from build123d import *

# Parameters (mm, degrees)
F0_R      = 73.025
F0_R_2    = 60.325
F1_DEPTH  = 69.85
F2_DEPTH  = 57.15
F3_SIZE   = 6.35
F4_DEPTH  = 12.7
F4_FACE_R = 73.025
F5_DEPTH  = 12.7


with BuildPart() as f1:
    # F0 (on Top) → F1 (new body)
    with BuildSketch(Plane.XY):
        Circle(F0_R)
        Circle(F0_R_2, mode=Mode.SUBTRACT)
        Circle(F0_R_2)
    extrude(amount=-F1_DEPTH)

    # F0 (on Top) → F2 (cut)
    with BuildSketch(Plane.XY):
        Circle(F0_R_2)
    extrude(amount=-F2_DEPTH, mode=Mode.SUBTRACT)

    # F3
    f3_edges = [f1.edges().sort_by_distance(p)[0] for p in [
        (-73.025, 0, -69.85),
    ]]
    chamfer(f3_edges, length=F3_SIZE)

    # F0 (on Top) → F4 (join)
    with BuildSketch(Plane.XY):
        Circle(F0_R_2)
        Circle(F0_R)
        Circle(F0_R_2, mode=Mode.SUBTRACT)
    extrude(amount=F4_DEPTH)

    # F4_face (on face) → F5 (join)
    with BuildSketch(Plane.XY.offset(12.7)):
        Circle(F4_FACE_R)
    extrude(amount=-F5_DEPTH)


solid = f1.part
Can you work these out from the model? Positions are in its coordinate system, mm. Round coordinates to 2 decimals unless told otherwise and drop trailing zeros. Loops run counter-clockwise (first coordinate to the right, second up) from the corner with the lowest first, then second, coordinate; pieces in that order, holes last. Notation, with made-up numbers: (-5, 0) - (54, 0) arc R10 ccw to (54, 8) - close; hole circle Ø2 at (-37.5, 49). An arc over 180 degrees is marked (long way). Write item = value, one per line. Start each with the question number.
(1) If we mould it in two halves opening along Y, with no side actions, what happens to faces 1 (the face through (-8.72, 66.413, -69.542)), 2 (the face through (-1, 1, -69.85)), 3 (the face through (-1, 1, 0))? For each: released by +Y, released by -Y, zero draft, split by the parting line, or undercut.
(2) For P1, Ø10, axis at x = -22.5, z = -57, coming from the -Y side; P2, Ø2, axis at y = -38.5, z = -42.5, coming from the -X side; P3, Ø1, axis at x = -21.5, z = -50, coming from the -Y side, each with a flat end and sliding along its axis, tell me the tip position at first contact or that it passes through.
(3) If we section it at C-C (z = -52.5): Please give me the cut outline in (x, y) (3 decimals).
(4) If we section it at A-A (x = 0): Please give me the cut outline in (y, z) (3 decimals).
(5) If I drill on probe 1 along Y at (x, z) = (0, -14) (3 decimals); probe 2 along Z at (x, y) = (22, 35); probe 3 along Y at (x, z) = (43, -57), over which ranges is the centre line in solid material (lowest first)? Write a range as [from, to].
Ans:
q1.face_1 = split by the parting line
q1.face_2 = zero draft
q1.face_3 = undercut
q2.P1 = -70.9
q2.P2 = -62.66
q2.P3 = -69.94
q3.outline = circle Ø146.05 at (0, 0); hole circle Ø120.65 at (0, 0)
q4.outline = (-73.025, -63.5) - (-66.675, -69.85) - (66.675, -69.85) - (73.025, -63.5) - (73.025, 12.7) - (-73.025, 12.7) - close; hole (-60.325, -57.15) - (60.325, -57.15) - (60.325, 0) - (-60.325, 0) - close
q5.probe_1 = [-73.025, -60.325], [60.325, 73.025]
q5.probe_2 = [-69.85, -57.15], [0, 12.7]
q5.probe_3 = [-59.02, -42.31], [42.31, 59.02]
